Could you check a few things on this model? Use its own coordinates, in mm. Face numbers are marked on the shaded views. Give positions to 0.01 mm unless a question says otherwise; leave off trailing zeros. Loops run counter-clockwise (first coordinate to the right, second up) from the corner with the lowest first, then second, coordinate; pieces in that order, holes last. Notation, with made-up numbers: (-29.5, 46) - (24.5, 46) arc R21 cw to (24.5, 61) - close; hole circle Ø5 at (66.25, -3.5). An arc over 180 degrees is marked (long way). Write each question's results on one line, items separated by ' | '. Start each with the question number.
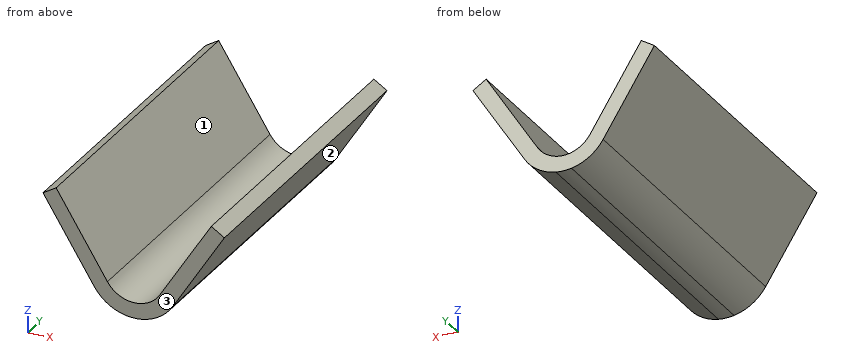
```python
from build123d import *

# Parameters (mm, degrees)
BOSS_EXTRUDE1_DEPTH    = 20
CONVERT_SOLID1_DEPTH   = 20
CONVERT_SOLID1_2_DEPTH = 20


# Read off the part's stored shape, not the designer's step: Convert-Solid1
with BuildPart() as part:
    # Sketch1 → Boss-Extrude1 (new body)
    with BuildSketch(Plane(origin=(0, 0, 0), x_dir=(1, 0, 0), z_dir=(0, 1, 0))):
        Polygon((0, 0), (5, 7.955252718), (10, 0), (11.693315732, 1.064275261), (5, 11.713678895), (-1.693315732, 1.064275261), align=None)
    extrude(amount=BOSS_EXTRUDE1_DEPTH)

    # Convert-Solid1 outline → Convert-Solid1 (cut)
    with BuildSketch(Plane(origin=(0, 0, 0), x_dir=(1, 0, 0), z_dir=(0, 1, 0))):
        with BuildLine():
            Line((5, 7.955252718), (5.503419817, 7.154286344))
            ThreePointArc((5.503419817, 7.154286344), (6.666935225, 6.69108534), (7.539973598, 5.793239432))
            Line((7.539973598, 5.793239432), (10.846657866, 0.53213763))
            Line((10.846657866, 0.53213763), (11.693315732, 1.064275261))
            Line((11.693315732, 1.064275261), (5, 11.713678895))
            Line((5, 11.713678895), (-1.693315732, 1.064275261))
            Line((-1.693315732, 1.064275261), (-0.846657866, 0.53213763))
            Line((-0.846657866, 0.53213763), (2.460026402, 5.793239432))
            ThreePointArc((2.460026402, 5.793239432), (3.333064775, 6.69108534), (4.496580183, 7.154286344))
            Line((4.496580183, 7.154286344), (5, 7.955252718))
        make_face()
    extrude(amount=CONVERT_SOLID1_DEPTH, mode=Mode.SUBTRACT)

    # Convert-Solid1 2 outline → Convert-Solid1 2 (add)
    with BuildSketch(Plane(origin=(0, 0, 0), x_dir=(1, 0, 0), z_dir=(0, 1, 0))):
        with BuildLine():
            ThreePointArc((3.306684268, 5.261101802), (5, 6.196826541), (6.693315732, 5.261101802))
            Line((6.693315732, 5.261101802), (5.503419817, 7.154286344))
            ThreePointArc((5.503419817, 7.154286344), (5, 7.196826541), (4.496580183, 7.154286344))
            Line((4.496580183, 7.154286344), (3.306684268, 5.261101802))
        make_face()
    extrude(amount=CONVERT_SOLID1_2_DEPTH)


solid = part.part
```
Q1. I want a section at D-D, the plane x = 4. List the corners of the cut face in (y, z) for me, then the cut area to 3 significant figures.
Q2. I need wall thicknesses on L1, parallel to X at y = 16.75, z = -5; L2, parallel to X at y = 2.5, z = -4; L3, parallel to Z at x = 1.25, y = 11.25. Which ranges of each line are inside material? Lowest first, please. Write a range as from..to.
Q3. I'm going to push flat-ended pins straight in: pin 1 Ø3 at (y, z) = (6.5, -2.5) entering from -X; pin 2 Ø5 at (x, y) = (8.5, 15.5) entering from +Z; pin 3 Ø4 at (y, z) = (15.5, -2) entering from -X; pin 4 Ø1.5 at (x, y) = (6, 6) entering from +Z. Where does each tip first touch, or does it pass through?
Q4. I want a section at C-C, the plane x = 1.5. List the corners of the cut face in (y, z) for me.
Q5. I want a section at B-B, the plane z = -4.5. List the corners of the cut face in (x, y) for me.
Q6. I want a section at A-A, the plane y = 9.25. List the corners of the cut face in (x, z) for me.
Q7. If we mould it in two halves opening along X, with no side actions, what happens to the marked faces 1, 2 and 3? For each: +X half, -X half, draft (parallel to the pull), parting line (faces both ways), or undercut.
Conclusion:
1) outline: (0, -7.03) - (20, -7.03) - (20, -5.93) - (0, -5.93) - close | area: 21.9 mm^2
2) L1: 1.96..3.14, 6.86..8.04 | L2: 1.33..2.51, 7.49..8.67 | L3: -3.87..-1.99
3) pin 1: x = -0.55 | pin 2: z = 0 | pin 3: x = -0.85 | pin 4: z = -5.17
4) outline: (0, -4.27) - (20, -4.27) - (20, -2.39) - (0, -2.39) - close
5) outline: (1.65, 0) - (2.83, 0) - (2.83, 20) - (1.65, 20) - close; (7.17, 0) - (8.35, 0) - (8.35, 20) - (7.17, 20) - close
6) outline: (-0.85, -0.53) - (2.46, -5.79) arc R3 ccw to (7.54, -5.79) - (10.85, -0.53) - (10, 0) - (6.69, -5.26) arc R2 cw to (3.31, -5.26) - (0, 0) - close
7) face 1: undercut | face 2: +X half | face 3: draft
